```python
from build123d import *

# Parameters (mm, degrees)
F1_DEPTH = 50.8


with BuildPart() as f1:
    # F0 (on Front) → F1 (new body)
    with BuildSketch(Plane.XZ):
        with BuildLine():
            ThreePointArc((-55.372, 136.61499), (0, 81.24299), (55.372, 136.61499))
            Line((55.372, 136.61499), (41.148, 136.61499))
            ThreePointArc((41.148, 136.61499), (0, 95.46699), (-41.148, 136.61499))
            Line((-41.148, 136.61499), (-55.372, 136.61499))
        make_face()
        with BuildLine():
            Line((41.148, 136.61499), (55.372, 136.61499))
            ThreePointArc((55.372, 136.61499), (0, 191.98699), (-55.372, 136.61499))
            Line((-55.372, 136.61499), (-41.148, 136.61499))
            ThreePointArc((-41.148, 136.61499), (0, 177.76299), (41.148, 136.61499))
        make_face()
        with BuildLine():
            ThreePointArc((-55.372, -136.61499), (0, -81.24299), (55.372, -136.61499))
            Line((55.372, -136.61499), (55.372, 136.61499))
            ThreePointArc((55.372, 136.61499), (0, 81.24299), (-55.372, 136.61499))
            Line((-55.372, 136.61499), (-55.372, -136.61499))
        make_face()
        with BuildLine():
            Line((41.148, -136.61499), (55.372, -136.61499))
            ThreePointArc((55.372, -136.61499), (0, -81.24299), (-55.372, -136.61499))
            Line((-55.372, -136.61499), (-41.148, -136.61499))
            ThreePointArc((-41.148, -136.61499), (0, -95.46699), (41.148, -136.61499))
        make_face()
        with BuildLine():
            ThreePointArc((-55.372, -136.61499), (0, -191.98699), (55.372, -136.61499))
            Line((55.372, -136.61499), (41.148, -136.61499))
            ThreePointArc((41.148, -136.61499), (0, -177.76299), (-41.148, -136.61499))
            Line((-41.148, -136.61499), (-55.372, -136.61499))
        make_face()
    extrude(amount=F1_DEPTH)


solid = f1.part
```
The listing builds one solid part. Answer for the finished solid, in the listing's coordinates (mm). Give positions to 0.01 mm unless a question says otherwise; leave off trailing zeros. Order: outer loops, then holes, each group sorted by start corner. A loop starts at its lowest first (then second) coordinate and runs counter-clockwise, first axis right, second up. Notation, with made-up numbers: (29.25, 21) -> (46.25, 21) arc R25 ccw to (46.25, 45) -> close; hole circle Ø2 at (40, -6.75). An arc over 180 degrees is marked (long way). Answer as a JSON object with one key per item and string values. Group by question number.
Item 1: The part is cut by section B-B on z = 128. Write down the section's boundary in (x, y).
Item 2: Determine the mould class of faces 1 (the cylindrical face through (-5.357, -25.044, -177.413)), 2 (the cylindrical face through (-1.218, -25.044, -191.974)), 3 (the cylindrical face through (1.218, -25.044, 191.974)) for opening direction Z: pulls with the +Z half, pulls with the -Z half, needs draft (parallel to the pull), parting line crosses it, or undercut.
Item 3: Flat-ended cylindrical pins translate along their axes: pin 1 (3 mm diameter, centred on y = -11, z = 140.5, fed in from +X); pin 2 (1 mm diameter, centred on x = 7.5, y = -38.5, fed in from -Z). Find the tip coordinate at first contact, or state that the pin passes through.
Item 4: The part is cut by section A-A on x = 0. Write down the section's boundary in (y, z), and give its area (3 significant figures).
Item 5: The part is cut by section C-C on y = -44. Write down the section's boundary in (x, z).
Item 6: Consider L1, parallel to Z at x = -2, y = -45.5; L2, parallel to Z at x = 0, y = -28.5; L3, parallel to X at y = -45, z = 110. Determine where each line is inside the solid, lowest interval first. Write a range as from..to.
Item 7: The part is cut by section D-D on x = -19. Write down the section's boundary in (y, z), and give its area (3 significant figures).
Result set:
{
 "1": {"outline": "(-55.37, -50.8) -> (-40.24, -50.8) -> (-40.24, 0) -> (-55.37, 0) -> close; (40.24, -50.8) -> (55.37, -50.8) -> (55.37, 0) -> (40.24, 0) -> close"},
 "2": {"face 1": "undercut", "face 2": "pulls with the -Z half", "face 3": "pulls with the +Z half"},
 "3": {"pin 1": "x = 55.32", "pin 2": "z = -191.54"},
 "4": {"outline": "(-50.8, -191.99) -> (0, -191.99) -> (0, -177.76) -> (-50.8, -177.76) -> close; (-50.8, -95.47) -> (0, -95.47) -> (0, 95.47) -> (-50.8, 95.47) -> close; (-50.8, 177.76) -> (0, 177.76) -> (0, 191.99) -> (-50.8, 191.99) -> close", "area": "11,100 mm²"},
 "5": {"outline": "(-55.37, -136.61) arc R55.37 ccw to (55.37, -136.61) -> (55.37, 136.61) arc R55.37 ccw to (-55.37, 136.61) -> close; hole circle Ø82.3 at (0, -136.61); hole circle Ø82.3 at (0, 136.61)"},
 "6": {"L1": "-191.95..-177.71, -95.52..95.52, 177.71..191.95", "L2": "-191.99..-177.76, -95.47..95.47, 177.76..191.99", "L3": "-55.37..-31.38, 31.38..55.37"},
 "7": {"outline": "(-50.8, -188.63) -> (0, -188.63) -> (0, -173.11) -> (-50.8, -173.11) -> close; (-50.8, -100.12) -> (0, -100.12) -> (0, 100.12) -> (-50.8, 100.12) -> close; (-50.8, 173.11) -> (0, 173.11) -> (0, 188.63) -> (-50.8, 188.63) -> close", "area": "11,700 mm²"}
}
